Design review of the part built by this model. Coordinates are the model's own, in mm. Face numbers are marked on the shaded views. A direction names the side the tool comes from. Round coordinates to 2 decimals unless told otherwise and drop trailing zeros. Order: outer loops, then holes, each group sorted by start corner. A loop starts at its lowest first (then second) coordinate and runs counter-clockwise, first axis right, second up. Notation, with made-up numbers: (30, 62) - (53, 62) arc R14 ccw to (53, 82) - close; hole circle Ø11 at (46, 49). An arc over 180 degrees is marked (long way). Write item = value, one per line.
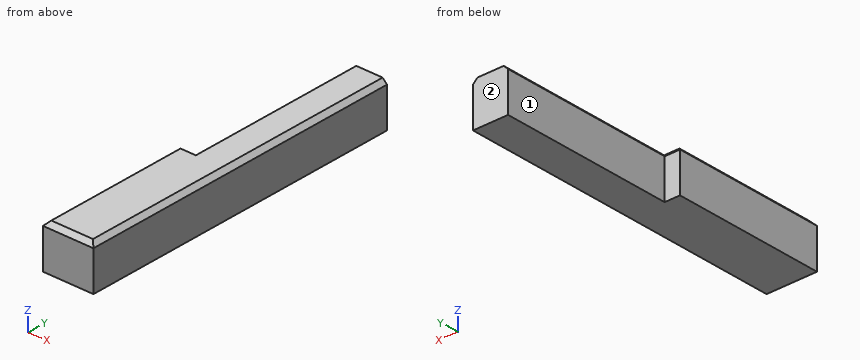
Autodesk Inventor part; units mm, degrees
ref_plane "YZ Plane" through (0, 0, 0) normal (1, 0, 0) x (0, 1, 0)
ref_plane "XZ Plane" through (0, 0, 0) normal (0, 1, 0) x (-1, 0, 0)
ref_plane "XY Plane" through (0, 0, 0) normal (0, 0, 1) x (1, 0, 0)
sketch "Sketch1" plane through (0, 0, 0) normal (0, 0, 1) x (1, 0, 0)
  line L0 (-11.5, -75) -> (11.5, -75)
  line L1 (11.5, -75) -> (11.5, 75)
  line L2 (11.5, 75) -> (-11.5, 75)
  line L3 (-11.5, 75) -> (-11.5, -75)
  line L4 (-11.5, -75) -> (11.5, 75) construction
  line L5 (11.5, -75) -> (-11.5, 75) construction
  line L6 (-11.5, 75) -> (-4.5, 75)
  line L7 (-4.5, 75) -> (-4.5, -5)
  line L8 (-4.5, -5) -> (-11.5, -5)
  line L9 (-11.5, -5) -> (-11.5, 75)
  point P0 (0, 0)
  dimension "d0" = 23
  dimension "d1" = 150
  dimension "d2" = 7
  dimension "d3" = 80
extrude "Extrusion1" add sketch "Sketch1" against normal blind 20 contours L3 L8 L7 L2 L1 L0
chamfer "Chamfer1" distance 2 angle 45 5 edges at (0, -75, 0) (-11.5, -40, 0) (11.5, 0, 0) (-8, -5, 0) (-4.5, 35, 0)
equation "\"d0\" = key_width"
equation "\"d1\" = key_length"
equation "\"d2\" = blackkey_halfwidth"
equation "\"d3\" = blackkey_length"
equation "\"d4\" = key_height"
properties part number "key_2"
Item 1: Take a section at B-B, the plane z = -16. State the section outline as (x, y) points.
Data:
outline = (-11.5, -75) - (11.5, -75) - (11.5, 75) - (-4.5, 75) - (-4.5, -5) - (-11.5, -5) - close
Item 2: Take a section at A-A, the plane x = -5.75. State the section outline as (y, z) points.
Data:
outline = (-75, -20) - (-5, -20) - (-5, -2) - (-7, 0) - (-73, 0) - (-75, -2) - close
Item 3: For the marked faces 1 and 2, list the 3-axis set-ups (+Z, -Z, +X, -X, +Y, -Y) from which the entire face can be reached by the end or side of a thin tool; tool diameter is ignored.
Data:
face_1 = +Z, -Z, -X, +Y
face_2 = +Z, -Z, +X, -X, +Y
Item 4: For line 1 along X through (y, z) = (65.5, -18); line 2 along Y through (x, z) = (-5.75, -6.5); line 3 along Y through (x, z) = (-9, -0.75), list the stretches that pass through material, from the lowest coordinate up. Write a range as [from, to].
Data:
line_1 = [-4.5, 11.5]
line_2 = [-75, -5]
line_3 = [-73.75, -6.25]
Item 5: Insertion check: P1, Ø5.5, axis at x = -8.5, z = -7, coming from the +Y side. The pin has a flat end and moves straight along its axis. Give the tip position at first contact, or say it passes through.
Data:
P1 = -5
